Model file for the job. Use its own axes, mm. Face numbers are marked on the shaded views. Round coordinates to 2 decimals unless told otherwise and drop trailing zeros. Order: outer loops, then holes, each group sorted by start corner. A loop starts at its lowest first (then second) coordinate and runs counter-clockwise, first axis right, second up. Notation, with made-up numbers: (88.25, -36) - (143.25, -36) arc R22 cw to (143.25, -15) - close; hole circle Ø9 at (-37.5, 67.25). An arc over 180 degrees is marked (long way). Put each result on its own line as item: value. Start each with the question number.
Item 1: Saw through at A-A on y = 8.5. List the corners of the cut face in (x, z).
Item 2: Saw through at B-B on y = 2.5. List the corners of the cut face in (x, z), plus the area to 3 significant figures.
Item 3: Mould opens along Z. For the marked faces 1, 2 and 3 say: pulls with the +Z half, pulls with the -Z half, needs draft (parallel to the pull), parting line crosses it, or undercut.
Item 4: Pin check, flat tips, straight feed: pin 1 Ø1 at (y, z) = (13.5, 25) entering from +X; pin 2 Ø2 at (x, y) = (23, 13) entering from +Z; pin 3 Ø6 at (x, y) = (41, 4.5) entering from -Z. Stop position of each tip, or through.
Item 5: Probe probe 1 along Z at (x, y) = (38, 7); probe 2 along Z at (x, y) = (32.5, 6.25); probe 3 along Z at (x, y) = (2.5, 4). List the from-to ranges inside material, lowest first.
Item 6: Saw through at C-C on x = -26. State how many separate pieces and enclosed holes the cut face has, plus the area to 3 significant figures.
```python
from build123d import *

# Parameters (mm, degrees)
SKETCH1_R                                           = 55
BOSS_EXTRUDE1_DEPTH                                 = 15.5
CBORE_FOR_M6_HEX_SOCKET_HEAD_CAP_SCREW1_D           = 18
CBORE_FOR_M6_HEX_SOCKET_HEAD_CAP_SCREW1_CBORE_D     = 25.5
CBORE_FOR_M6_HEX_SOCKET_HEAD_CAP_SCREW1_CBORE_DEPTH = 3.5
SKETCH5_R                                           = 13
CUT_EXTRUDE1_DEPTH                                  = 3
F_5_0MM_DOWEL_HOLE1_D                               = 5
CHAMFER1_SIZE                                       = 1
CHAMFER2_SIZE                                       = 1
CBORE_FOR_M5_HEX_SOCKET_HEAD_CAP_SCREW1_D           = 5.5
CBORE_FOR_M5_HEX_SOCKET_HEAD_CAP_SCREW1_CBORE_D     = 9
CBORE_FOR_M5_HEX_SOCKET_HEAD_CAP_SCREW1_CBORE_DEPTH = 6


with BuildPart() as part:
    # Sketch1 → Boss-Extrude1 (new body)
    with BuildSketch(Plane(origin=(0, 0, 0), x_dir=(1, 0, 0), z_dir=(0, 1, 0))):
        with Locations(Location((0, 0, 0), (0, 0, 270))):
            Circle(SKETCH1_R)
    extrude(amount=BOSS_EXTRUDE1_DEPTH)

    # CBORE for M6 Hex Socket Head Cap Screw1 (through all)
    with Locations(Plane(origin=(0, 15.5, 0), x_dir=(1, 0, 0), z_dir=(0, 1, 0))):
        with Locations((-32.5, 21), (32.5, 21), (32.5, -21), (-32.5, -21)):
            CounterBoreHole(CBORE_FOR_M6_HEX_SOCKET_HEAD_CAP_SCREW1_D / 2, CBORE_FOR_M6_HEX_SOCKET_HEAD_CAP_SCREW1_CBORE_D / 2, CBORE_FOR_M6_HEX_SOCKET_HEAD_CAP_SCREW1_CBORE_DEPTH)

    # Sketch5 → Cut-Extrude1 (cut)
    with BuildSketch(Plane(origin=(0, 15.5, 0), x_dir=(1, 0, 0), z_dir=(0, 1, 0))):
        with Locations(Location((0, 0, 0), (0, 0, 270))):
            Circle(SKETCH5_R)
    extrude(amount=-CUT_EXTRUDE1_DEPTH, mode=Mode.SUBTRACT)

    # Ø5.0mm Dowel Hole1 (through all)
    with Locations(Plane(origin=(0, 12.5, 0), x_dir=(1, 0, 0), z_dir=(0, 1, 0))):
        with Locations((-8, 0), (8, 0)):
            Hole(F_5_0MM_DOWEL_HOLE1_D / 2)

    # Chamfer1
    chamfer1_edges = [part.edges().sort_by_distance(p)[0] for p in [
        (0, 15.5, -13),
        (0, 15.5, -55),
    ]]
    chamfer(chamfer1_edges, length=CHAMFER1_SIZE)

    # Chamfer2
    chamfer2_edges = [part.edges().sort_by_distance(p)[0] for p in [
        (0, 0, -55),
    ]]
    chamfer(chamfer2_edges, length=CHAMFER2_SIZE)

    # CBORE for M5 Hex Socket Head Cap Screw1 (through all)
    with Locations(Plane(origin=(0, 0, 0), x_dir=(-1, 0, 0), z_dir=(0, -1, 0))):
        with Locations((0, 0)):
            CounterBoreHole(CBORE_FOR_M5_HEX_SOCKET_HEAD_CAP_SCREW1_D / 2, CBORE_FOR_M5_HEX_SOCKET_HEAD_CAP_SCREW1_CBORE_D / 2, CBORE_FOR_M5_HEX_SOCKET_HEAD_CAP_SCREW1_CBORE_DEPTH)


solid = part.part
```
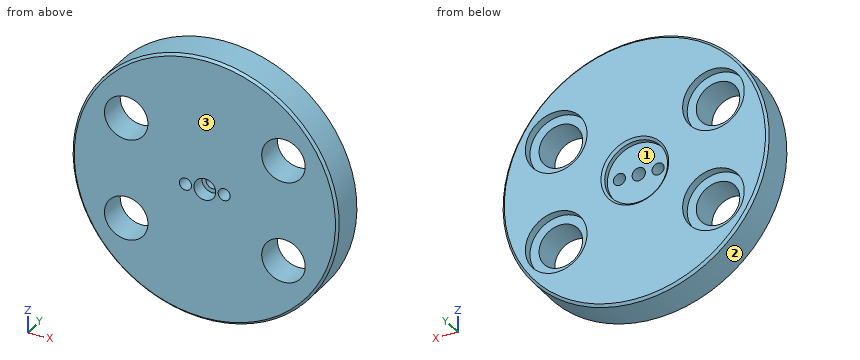
Results found:
1. outline: circle Ø110 at (0, 0); hole circle Ø18 at (-32.5, -21); hole circle Ø18 at (-32.5, 21); hole circle Ø5 at (-8, 0); hole circle Ø5.5 at (0, 0); hole circle Ø5 at (8, 0); hole circle Ø18 at (32.5, -21); hole circle Ø18 at (32.5, 21)
2. outline: circle Ø110 at (0, 0); hole circle Ø18 at (-32.5, -21); hole circle Ø18 at (-32.5, 21); hole circle Ø5 at (-8, 0); hole circle Ø9 at (0, 0); hole circle Ø5 at (8, 0); hole circle Ø18 at (32.5, -21); hole circle Ø18 at (32.5, 21)
2. area: 8,380 mm²
3. face 1: undercut
3. face 2: parting line crosses it
3. face 3: needs draft
4. pin 1: stops at x = 49.24
4. pin 2: stops at z = 50.41
4. pin 3: stops at z = -39.76
5. probe 1: z = -39.76 to -28.12, -13.88 to 13.88, 28.12 to 39.76
5. probe 2: z = -44.37 to -30, -12 to 12, 30 to 44.37
5. probe 3: z = -54.94 to -3.74, 3.74 to 54.94
6. separate pieces: 3
6. enclosed holes: 0
6. area: 1,050 mm²
